The listing builds one solid part. Answer for the finished solid, in the listing's coordinates (mm). Face numbers are marked on the shaded views. Give positions to 0.01 mm unless a question says otherwise; leave off trailing zeros. Order: outer loops, then holes, each group sorted by start corner. A loop starts at its lowest first (then second) coordinate and runs counter-clockwise, first axis right, second up.
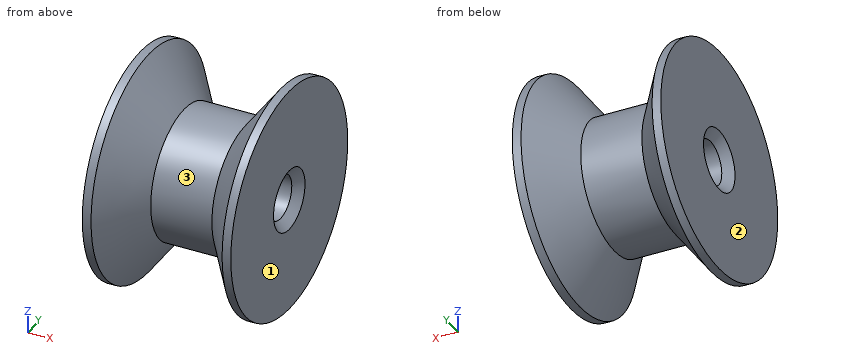
```python
from build123d import *

# Parameters (mm, degrees)
F2_SIZE2 = 10.99999
F2_SIZE  = 7.99999
F3_SIZE  = 2


# Not quite as in the source:
# - a fillet or chamfer is up to 0.001 mm smaller than in the source, because OpenCascade refuses the exact size


with BuildPart() as f1:
    # F0 (on Front) → F1 (revolve)
    with BuildSketch(Plane.XZ):
        Polygon((0, 26), (0, 5), (34, 5), (34, 26), (32, 26), (32, 15), (2, 15), (2, 26), align=None)
    revolve(axis=Axis((17, 0, 0), (1, 0, 0)))

    # F2 (size 8 and 11 in the source; OpenCascade refuses exactly that, so slightly less here)
    f2_edges = [f1.edges().sort_by_distance(p)[0] for p in [
        (2, 0, -15),
        (32, 0, -15),
    ]]
    f2_side = f1.faces().sort_by_distance((17, 0, -15))[0]
    chamfer(f2_edges, length=F2_SIZE, length2=F2_SIZE2, reference=f2_side)

    # F3
    f3_edges = [f1.edges().sort_by_distance(p)[0] for p in [
        (0, 0, -5),
        (34, 0, -5),
    ]]
    chamfer(f3_edges, length=F3_SIZE)


solid = f1.part
```
1) Straight lines are drawn through the part: probe 1 along Z at (x, y) = (20, 0); probe 2 along X at (y, z) = (4.5, -19). For each, find the intervals that lie inside material, in ascending order.
Geometry says:
probe 1: z = -15 to -5, 5 to 15
probe 2: x = 0 to 6.71, 27.29 to 34
2) For a pull along X with two mould halves and no side action, classify the marked faces 1, 2 and 3 as +X half, -X half, draft (parallel to the pull), parting line (faces both ways), or undercut.
Geometry says:
face 1: +X half
face 2: -X half
face 3: undercut
3) Given P1, Ø5, axis at x = 22, z = 4.5, coming from the +Y side; P2, Ø2, axis at x = 25, y = 18.5, coming from the +Z side; P3, Ø8, axis at x = 8, y = 12.5, coming from the +Z side; P4, Ø12, axis at x = 28.5, y = 12, coming from the +Z side, each flat-ended and moving along its own axis, determine where each tip first touches the part or whether it passes through.
Geometry says:
P1: stops at y = 15.1
P2: passes through
P3: stops at z = 20.03
P4: stops at z = 25
4) Find section D-D (x = 27). Write down the section's boundary in (y, z).
Geometry says:
outline: circle Ø38.25 at (0, 0); hole circle Ø10 at (0, 0)
5) Find section C-C (x = 21). Write down the section's boundary in (y, z), then the cut area to 3 significant figures.
Geometry says:
outline: circle Ø30 at (0, 0); hole circle Ø10 at (0, 0)
area: 628 mm2
